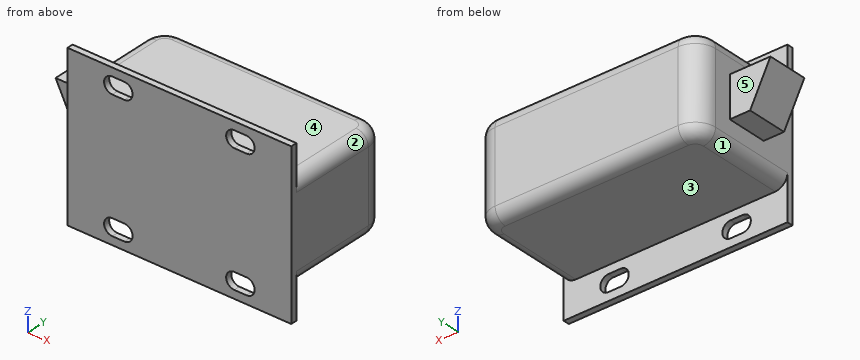
from build123d import *

# Parameters (mm, degrees)
SKETCH1_W           = 55
SKETCH1_H           = 39.5
BOSS_EXTRUDE1_DEPTH = 27.7
SKETCH2_W           = 8
SKETCH2_H           = 26.2
CUT_EXTRUDE1_DEPTH  = 65.877365082
SKETCH3_W           = 8
SKETCH3_H           = 26.2
CUT_EXTRUDE2_DEPTH  = 65.877365082
CUT_EXTRUDE3_DEPTH  = 50.345111207
CUT_EXTRUDE4_DEPTH  = 51.15765146
CUT_EXTRUDE5_DEPTH  = 50.345111207
CUT_EXTRUDE6_DEPTH  = 51.15765146
BOSS_EXTRUDE2_DEPTH = 10
FILLET1_R           = 5
FILLET2_R           = 3


with BuildPart() as part:
    # Sketch1 → Boss-Extrude1 (new body)
    with BuildSketch(Plane(origin=(0, 13.85, 0), x_dir=(1, 0, 0), z_dir=(0, 1, 0))):
        with Locations((0, -11.75)):
            Rectangle(SKETCH1_W, SKETCH1_H)
    extrude(amount=-BOSS_EXTRUDE1_DEPTH)

    # Sketch2 → Cut-Extrude1 (cut, through all)
    with BuildSketch(Plane.ZY.offset(27.5)):
        with Locations((27.5, 0.75)):
            Rectangle(SKETCH2_W, SKETCH2_H)
    extrude(amount=-CUT_EXTRUDE1_DEPTH, mode=Mode.SUBTRACT)

    # Sketch3 → Cut-Extrude2 (cut, through all)
    with BuildSketch(Plane.ZY.offset(27.5)):
        with Locations((-4, 0.75)):
            Rectangle(SKETCH3_W, SKETCH3_H)
    extrude(amount=-CUT_EXTRUDE2_DEPTH, mode=Mode.SUBTRACT)

    # Sketch4 → Cut-Extrude3 (cut, through all)
    with BuildSketch(Plane(origin=(0, -12.35, 0), x_dir=(-1, 0, 0), z_dir=(0, 1, 0))):
        with BuildLine():
            Line((-13.5, -2), (-16.5, -2))
            ThreePointArc((-16.5, -2), (-18.5, -4), (-16.5, -6))
            Line((-16.5, -6), (-13.5, -6))
            ThreePointArc((-13.5, -6), (-11.5, -4), (-13.5, -2))
        make_face()
    extrude(amount=-CUT_EXTRUDE3_DEPTH, mode=Mode.SUBTRACT)

    # Sketch5 → Cut-Extrude4 (cut, through all)
    with BuildSketch(Plane.XZ.offset(13.85)):
        with BuildLine():
            Line((-16.5, -6), (-13.5, -6))
            ThreePointArc((-13.5, -6), (-11.5, -4), (-13.5, -2))
            Line((-13.5, -2), (-16.5, -2))
            ThreePointArc((-16.5, -2), (-18.5, -4), (-16.5, -6))
        make_face()
    extrude(amount=-CUT_EXTRUDE4_DEPTH, mode=Mode.SUBTRACT)

    # Sketch6 → Cut-Extrude5 (cut, through all)
    with BuildSketch(Plane(origin=(0, -12.35, 0), x_dir=(-1, 0, 0), z_dir=(0, 1, 0))):
        with BuildLine():
            Line((16.5, 29.5), (13.5, 29.5))
            ThreePointArc((13.5, 29.5), (11.5, 27.5), (13.5, 25.5))
            Line((13.5, 25.5), (16.5, 25.5))
            ThreePointArc((16.5, 25.5), (18.5, 27.5), (16.5, 29.5))
        make_face()
    extrude(amount=-CUT_EXTRUDE5_DEPTH, mode=Mode.SUBTRACT)

    # Sketch7 → Cut-Extrude6 (cut, through all)
    with BuildSketch(Plane.XZ.offset(13.85)):
        with BuildLine():
            Line((13.5, 25.5), (16.5, 25.5))
            ThreePointArc((16.5, 25.5), (18.5, 27.5), (16.5, 29.5))
            Line((16.5, 29.5), (13.5, 29.5))
            ThreePointArc((13.5, 29.5), (11.5, 27.5), (13.5, 25.5))
        make_face()
    extrude(amount=-CUT_EXTRUDE6_DEPTH, mode=Mode.SUBTRACT)

    # Sketch8 → Boss-Extrude2 (add)
    with BuildSketch(Plane.XZ.offset(5.35)):
        Polygon((-37.5, 16.75), (-32.5, 6.75), (-27.5, 6.75), (-27.5, 16.75), align=None)
    extrude(amount=-BOSS_EXTRUDE2_DEPTH)

    # Fillet1
    fillet1_edges = [part.edges().sort_by_distance(p)[0] for p in [
        (27.5, 13.85, 11.75),
        (-27.5, 13.85, 11.75),
    ]]
    fillet(fillet1_edges, radius=FILLET1_R)

    # Fillet2
    fillet2_edges = [part.edges().sort_by_distance(p)[0] for p in [
        (0, 13.85, 0),
        (0, 13.85, 23.5),
        (-26.035533906, 12.385533906, 0),
        (26.035533906, 12.385533906, 0),
        (27.5, -1.75, 23.5),
        (-27.5, -1.75, 23.5),
        (-26.035533906, 12.385533906, 23.5),
        (26.035533906, 12.385533906, 23.5),
        (27.5, -1.75, 0),
        (-27.5, -1.75, 0),
    ]]
    fillet(fillet2_edges, radius=FILLET2_R)


solid = part.part
Verification items for the finished model (mm, model axes). Face numbers are marked on the shaded views. A direction names the side the tool comes from. Round coordinates to 2 decimals unless told otherwise and drop trailing zeros. Write each loop counter-clockwise with the first axis right and the second up, starting at its lowest first coordinate (ties: lowest second). Pieces come first, ordered by that corner, then holes.
(1) Depth check by flat-ended pin: pin 1 Ø4 at (x, y) = (-17, 9.5) entering from +Z; pin 2 Ø9 at (x, z) = (9, -3) entering from +Y; pin 3 Ø3 at (y, z) = (1, 13.5) entering from -X (3 decimals). Enter the tip coordinate at first touch or a pass-through.
Returned:
pin 1: stops at z = 23.5
pin 2: stops at y = 13.45
pin 3: stops at x = -36.625
(2) Section check D-D (z = 18). Enter the section's corners in (x, y), plus the area to 3 significant figures.
Returned:
outline: (-27.5, -13.85) - (27.5, -13.85) - (27.5, 8.85) arc R5 ccw to (22.5, 13.85) - (-22.5, 13.85) arc R5 ccw to (-27.5, 8.85) - close
area: 1,510 mm2
(3) Access from +Z, -Z, +X, -X, +Y, -Y to the whole of each face (thin tool, end or side, straight path). Record for the marked faces 1, 2, 3, 4 and 5.
Returned:
face 1: -Z, -X, +Y
face 2: +Z, +X, +Y
face 3: -Z, +X, -X, +Y
face 4: +Z, +X, -X, +Y
face 5: +Z, -Z, -X, +Y
(4) Section check A-A (z = -4). Enter the section's corners in (x, y).
Returned:
outline: (-27.5, -13.85) - (-18.5, -13.85) - (-18.5, -12.35) - (-27.5, -12.35) - close; (-11.5, -13.85) - (11.5, -13.85) - (11.5, -12.35) - (-11.5, -12.35) - close; (18.5, -13.85) - (27.5, -13.85) - (27.5, -12.35) - (18.5, -12.35) - close
(5) Material ranges on line 1 (X direction, y = -4.5, z = 17); line 2 (Z direction, x = -1.5, y = -3.75); line 3 (Y direction, x = 11.5, z = -0.5), recorded low to high.
Returned:
line 1: x = -27.5 to 27.5
line 2: z = 0 to 23.5
line 3: y = -13.85 to -12.35
(6) Section check C-C (x = 20). Enter the section's corners in (y, z), plus the area to 3 significant figures.
Returned:
outline: (-13.85, -8) - (-12.35, -8) - (-12.35, 0) - (10.85, 0) arc R3 ccw to (13.85, 3) - (13.85, 20.5) arc R3 ccw to (10.85, 23.5) - (-12.35, 23.5) - (-12.35, 31.5) - (-13.85, 31.5) - close
area: 671 mm2
(7) Section check B-B (y = 3.5). Enter the section's corners in (x, z).
Returned:
outline: (-37.5, 16.75) - (-32.5, 6.75) - (-27.5, 6.75) - (-27.5, 3) arc R3 ccw to (-24.5, 0) - (24.5, 0) arc R3 ccw to (27.5, 3) - (27.5, 20.5) arc R3 ccw to (24.5, 23.5) - (-24.5, 23.5) arc R3 ccw to (-27.5, 20.5) - (-27.5, 16.75) - close
